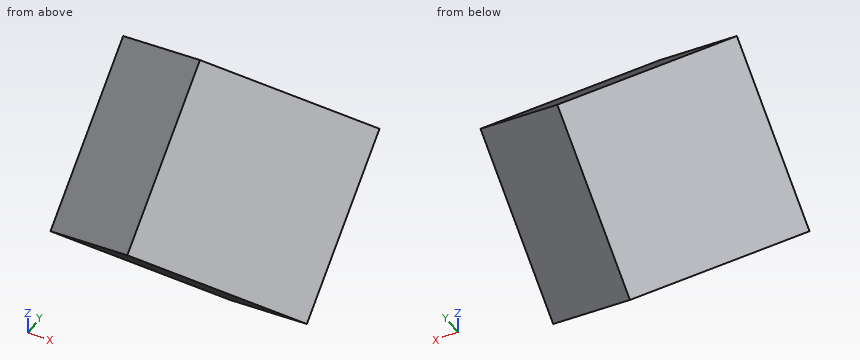
from build123d import *

# Parameters (mm, degrees)
F1_W     = 50
F1_H     = 50
F2_DEPTH = 25
F4_ANGLE = 45
F6_ANGLE = 45


with BuildPart() as f2:
    # F1 (on Top) → F2 (new body, symmetric)
    with BuildSketch(Plane.XY):
        Rectangle(F1_W, F1_H)
    extrude(amount=F2_DEPTH, both=True)


with BuildPart() as f2_1:
    # F4: moved
    add(f2.part.rotate(Axis((0, 0, 0), (0, 1, 0)), F4_ANGLE))


with BuildPart() as f2_2:
    # F6: moved
    add(f2_1.part.rotate(Axis((0, 0, 0), (1, 0, 0)), F6_ANGLE))


solid = f2_2.part
The listing builds one solid part. Answer for the finished solid, in the listing's coordinates (mm). Give positions to 0.01 mm unless a question says otherwise; leave off trailing zeros. Loops run counter-clockwise (first coordinate to the right, second up) from the corner with the lowest first, then second, coordinate; pieces in that order, holes last. Notation, with made-up numbers: (78.25, 64) - (131.25, 64) arc R37 ccw to (131.25, 100) - close; hole circle Ø10 at (7, 10). An arc over 180 degrees is marked (long way). Write each question's results on one line, items separated by ' | '.
1. Find section A-A, the plane y = -6. Write down the section's boundary in (x, z).
Resolved:
outline: (-35.36, -6) - (-18.84, -29.36) - (18.84, -29.36) - (35.36, -6) - (1.87, 41.36) - (-1.87, 41.36) - close
2. Flat-ended cylindrical pins translate along their axes: P1, Ø10, axis at x = 11.5, z = -23.5, coming from the +Y side; P2, Ø6, axis at x = 11, z = 25.5, coming from the -Y side; P3, Ø5, axis at x = -12, y = -6.5, coming from the -Z side. Find the tip coordinate at first contact, or state that the pin passes through.
Resolved:
P1: stops at y = 18.9 | P2: stops at y = -14.14 | P3: stops at z = -31.36
3. Find section B-B, the plane z = -9. Write down the section's boundary in (x, y).
Resolved:
outline: (-35.36, -9) - (-23.08, -26.36) - (23.08, -26.36) - (35.36, -9) - (0, 41) - close
4. Find section C-C, the plane x = 15.5. Write down the section's boundary in (y, z), then the cut area to 3 significant figures.
Resolved:
outline: (-31.72, -3.64) - (-3.64, -31.72) - (31.72, 3.64) - (3.64, 31.72) - close | area: 1,990 mm^2
5. Consider probe 1 along Z at (x, y) = (-18, 0.5); probe 2 along Y at (x, z) = (13, 13); probe 3 along X at (y, z) = (-8, 2). Determine where each line is inside the solid, lowest interval first. Write a range as from..to.
Resolved:
probe 1: z = -24.04..25.04 | probe 2: y = -18.62..22.36 | probe 3: x = -28.28..28.28
6. Find section D-D, the plane z = 2.5. Write down the section's boundary in (x, y).
Resolved:
outline: (-35.36, 2.5) - (-6.82, -37.86) - (6.82, -37.86) - (35.36, 2.5) - (13.89, 32.86) - (-13.89, 32.86) - close
